The listing builds one solid part. Answer for the finished solid, in the listing's coordinates (mm). A direction names the side the tool comes from. Give positions to 0.01 mm unless a question says otherwise; leave off trailing zeros. Order: outer loops, then holes, each group sorted by start corner. A loop starts at its lowest first (then second) coordinate and runs counter-clockwise, first axis right, second up.
```python
from build123d import *

# Parameters (mm, degrees)
SKETCH_1_R          = 6
EXTRUDE_1_DEPTH     = 4
SKETCH_2_R          = 6.75
EXTRUDE_2_DEPTH     = 1
SKETCH_3_R          = 4
CUT_EXTRUDE_1_DEPTH = 5
SKETCH_4_R          = 5.5
SKETCH_4_R_2        = 4.5
CUT_EXTRUDE_2_DEPTH = 0.2
SKETCH_5_R          = 5.5
SKETCH_5_R_2        = 4.5
CUT_EXTRUDE_3_DEPTH = 0.2
FILLET_1_R          = 0.1


with BuildPart() as part:
    # 草圖1 → 填料-伸長1 (new body)
    with BuildSketch(Plane.XY):
        Circle(SKETCH_1_R)
    extrude(amount=EXTRUDE_1_DEPTH)

    # 草圖2 → 填料-伸長2 (add)
    with BuildSketch(Plane.XY.offset(4)):
        Circle(SKETCH_2_R)
    extrude(amount=-EXTRUDE_2_DEPTH)

    # 草圖3 → 除料-伸長1 (cut, through all)
    with BuildSketch(Plane(origin=(0, 0, 0), x_dir=(-1, 0, 0), z_dir=(0, 0, -1))):
        Circle(SKETCH_3_R)
    extrude(amount=-CUT_EXTRUDE_1_DEPTH, mode=Mode.SUBTRACT)

    # 草圖4 → 除料-伸長2 (cut)
    with BuildSketch(Plane(origin=(0, 0, 0), x_dir=(-1, 0, 0), z_dir=(0, 0, -1))):
        Circle(SKETCH_4_R)
        Circle(SKETCH_4_R_2, mode=Mode.SUBTRACT)
    extrude(amount=-CUT_EXTRUDE_2_DEPTH, mode=Mode.SUBTRACT)

    # 草圖5 → 除料-伸長3 (cut)
    with BuildSketch(Plane.XY.offset(4)):
        Circle(SKETCH_5_R)
        Circle(SKETCH_5_R_2, mode=Mode.SUBTRACT)
    extrude(amount=-CUT_EXTRUDE_3_DEPTH, mode=Mode.SUBTRACT)

    # 圓角1
    fillet_1_edges = [part.edges().sort_by_distance(p)[0] for p in [
        (-6, 0, 0),
    ]]
    fillet(fillet_1_edges, radius=FILLET_1_R)


solid = part.part
```
1) A tool of negligible diameter and unlimited length cuts with its end or side. For faces 1 (the flat face through (-5, -4, 3)), 2 (the cylindrical face through (-1.46, -6.59, 3.51)), 3 (the flat face through (-5, 0, 3.8)), from which of +Z, -Z, +X, -X, +Y, -Y can it reach the whole face along a straight path? Write none if from no direction.
Geometry says:
face 1: -Z
face 2: +Z, -Z
face 3: +Z
2) Find section D-D (z = 3.45). Write down the section's boundary in (x, y), then the cut area to 3 significant figures.
Geometry says:
outline: circle Ø13.5 at (0, 0); hole circle Ø8 at (0, 0)
area: 92.9 mm2
3) For a pull along Y with two mould halves and no side action, classify faces 4 (the cylindrical face through (-6, 0, 2)), 5 (the flat face through (5, 0, 0.2)), 6 (the flat face through (-6, 0, 4)) as +Y half, -Y half, draft (parallel to the pull), parting line (faces both ways), or undercut.
Geometry says:
face 4: parting line
face 5: undercut
face 6: draft
4) Straight lines are drawn through the part: probe 1 along Y at (x, z) = (0, 3.9); probe 2 along Y at (x, z) = (0, 1.6); probe 3 along Y at (x, z) = (0, 0.1). For each, find the intervals that lie inside material, in ascending order.
Geometry says:
probe 1: y = -6.75 to -5.5, -4.5 to -4, 4 to 4.5, 5.5 to 6.75
probe 2: y = -6 to -4, 4 to 6
probe 3: y = -6 to -5.5, -4.5 to -4, 4 to 4.5, 5.5 to 6
5) Given P1, Ø7, axis at x = 3.5, y = 1.5, coming from the -Z side; P2, Ø2, axis at x = 2, z = 3, coming from the -Y side, each flat-ended and moving along its own axis, determine where each tip first touches the part or whether it passes through.
Geometry says:
P1: stops at z = 0
P2: stops at y = -6.68
6) Find section C-C (z = 2.55). Write down the section's boundary in (x, y), then the cut area to 3 significant figures.
Geometry says:
outline: circle Ø12 at (0, 0); hole circle Ø8 at (0, 0)
area: 62.8 mm2
